Part model, mm, in its own coordinate system. A direction names the side the tool comes from. Round coordinates to 2 decimals unless told otherwise and drop trailing zeros. Order: outer loops, then holes, each group sorted by start corner. A loop starts at its lowest first (then second) coordinate and runs counter-clockwise, first axis right, second up. Notation, with made-up numbers: (11, -39.75) -> (36, -39.75) arc R27 cw to (36, -14.75) -> close; hole circle Ø8 at (29, 52). An arc over 180 degrees is marked (long way). Return JSON: item names as keys, results as strings. Group by question number.
from build123d import *

# Parameters (mm, degrees)
SKETCH1_W           = 42.3
SKETCH1_H           = 42.3
SKETCH1_R           = 2.5
BOSS_EXTRUDE1_DEPTH = 42.3
SKETCH2_R           = 2.5
BOSS_EXTRUDE2_DEPTH = 24
SKETCH3_R           = 7.5
BOSS_EXTRUDE3_DEPTH = 2
SKETCH4_W           = 15
SKETCH4_H           = 42.3
CUT_EXTRUDE1_DEPTH  = 1
SKETCH5_W           = 41.3
SKETCH5_H           = 15
CUT_EXTRUDE2_DEPTH  = 1


with BuildPart() as part:
    # Sketch1 → Boss-Extrude1 (new body)
    with BuildSketch(Plane.XY):
        Rectangle(SKETCH1_W, SKETCH1_H)
        with Locations((-15.5, 15.5)):
            Circle(SKETCH1_R, mode=Mode.SUBTRACT)
        with Locations((15.5, 15.5)):
            Circle(SKETCH1_R, mode=Mode.SUBTRACT)
        with Locations((15.5, -15.5)):
            Circle(SKETCH1_R, mode=Mode.SUBTRACT)
        with Locations((-15.5, -15.5)):
            Circle(SKETCH1_R, mode=Mode.SUBTRACT)
    extrude(amount=BOSS_EXTRUDE1_DEPTH)

    # Sketch2 → Boss-Extrude2 (add)
    with BuildSketch(Plane.XY.offset(42.3)):
        Circle(SKETCH2_R)
    extrude(amount=BOSS_EXTRUDE2_DEPTH)

    # Sketch3 → Boss-Extrude3 (add)
    with BuildSketch(Plane.XY.offset(42.3)):
        Circle(SKETCH3_R)
    extrude(amount=BOSS_EXTRUDE3_DEPTH)

    # Sketch4 → Cut-Extrude1 (cut)
    with BuildSketch(Plane(origin=(21.15, 0, 0), x_dir=(0, 0, -1), z_dir=(1, 0, 0))):
        with Locations((-21.15, 0)):
            Rectangle(SKETCH4_W, SKETCH4_H)
    cut_extrude1 = extrude(amount=-CUT_EXTRUDE1_DEPTH, mode=Mode.SUBTRACT)

    # Sketch5 → Cut-Extrude2 (cut)
    with BuildSketch(Plane(origin=(0, 21.15, 0), x_dir=(1, 0, 0), z_dir=(0, 1, 0))):
        with Locations((-0.5, -21.15)):
            Rectangle(SKETCH5_W, SKETCH5_H)
    extrude(amount=-CUT_EXTRUDE2_DEPTH, mode=Mode.SUBTRACT)

    # Mirror1: Cut-Extrude1 across plane
    add(cut_extrude1.mirror(Plane(origin=(0, 0, 0), x_dir=(0, 0, 1), z_dir=(1, 0, 0))), mode=Mode.SUBTRACT)


solid = part.part
(1) Saw through at C-C, the plane x = 14. List the corners of the cut face in (y, z), and give its area (3 significant figures).
(2) Pin check, flat tips, straight feed: P1, Ø4, axis at x = 15.5, y = -15.5, coming from the +Z side; P2, Ø4.5, axis at y = 5, z = 18.5, coming from the -X side; P3, Ø7.5, axis at x = 2, z = 20.5, coming from the +Y side; P4, Ø1, axis at x = 9, y = 7.5, coming from the +Z side. Stop position of each tip, or through.
(3) Tool access for faces 1 (the cylindrical face through (-7.493, 0.33, 43.286)), 2 (the flat face through (-21.15, 0, 7)): list every direction of +Z, -Z, +X, -X, +Y, -Y with a clear straight run to the whole face (end or side of a thin tool).
(4) Mould opens along Z. For faces 3 (the flat face through (0, 0, 0)), 4 (the flat face through (-0.1, 20.5, 13.65)), 5 (the cylindrical face through (-0.54, -2.44, 55.15)), 6 (the flat face through (20.15, 0, 21)) say: pulls with the +Z half, pulls with the -Z half, needs draft (parallel to the pull), parting line crosses it, or undercut.
(5) Saw through at D-D, the plane x = 0. List the corners of the cut face in (y, z).
(6) Saw through at B-B, the plane y = 15.5. List the corners of the cut face in (x, z).
(7) Saw through at A-A, the plane z = 32. List the corners of the cut face in (x, y), and give its area (3 significant figures).
(8) Probe L1, parallel to Y at x = -15.5, z = 17.5; L2, parallel to Y at x = -15, z = 17; L3, parallel to X at y = 15, z = 15. List the from-to ranges inside material, lowest first. Write a range as [from, to].
Results are:
{
 "1": {"outline": "(-21.15, 0) -> (-17.5, 0) -> (-17.5, 42.3) -> (-21.15, 42.3) -> close; (-13.5, 0) -> (13.5, 0) -> (13.5, 42.3) -> (-13.5, 42.3) -> close; (17.5, 0) -> (21.15, 0) -> (21.15, 13.65) -> (20.15, 13.65) -> (20.15, 28.65) -> (21.15, 28.65) -> (21.15, 42.3) -> (17.5, 42.3) -> close", "area": "1,440 mm^2"},
 "2": {"P1": "passes through", "P2": "stops at x = -20.15", "P3": "stops at y = 20.15", "P4": "stops at z = 42.3"},
 "3": {"face 1": "+Z", "face 2": "+Z, -Z, -X, +Y, -Y"},
 "4": {"face 3": "pulls with the -Z half", "face 4": "undercut", "face 5": "needs draft", "face 6": "undercut"},
 "5": {"outline": "(-21.15, 0) -> (21.15, 0) -> (21.15, 13.65) -> (20.15, 13.65) -> (20.15, 28.65) -> (21.15, 28.65) -> (21.15, 42.3) -> (7.5, 42.3) -> (7.5, 44.3) -> (2.5, 44.3) -> (2.5, 66.3) -> (-2.5, 66.3) -> (-2.5, 44.3) -> (-7.5, 44.3) -> (-7.5, 42.3) -> (-21.15, 42.3) -> close"},
 "6": {"outline": "(-21.15, 0) -> (-18, 0) -> (-18, 42.3) -> (-21.15, 42.3) -> (-21.15, 28.65) -> (-20.15, 28.65) -> (-20.15, 13.65) -> (-21.15, 13.65) -> close; (-13, 0) -> (13, 0) -> (13, 42.3) -> (-13, 42.3) -> close; (18, 0) -> (21.15, 0) -> (21.15, 13.65) -> (20.15, 13.65) -> (20.15, 28.65) -> (21.15, 28.65) -> (21.15, 42.3) -> (18, 42.3) -> close"},
 "7": {"outline": "(-21.15, -21.15) -> (21.15, -21.15) -> (21.15, 21.15) -> (-21.15, 21.15) -> close; hole circle Ø5 at (-15.5, -15.5); hole circle Ø5 at (-15.5, 15.5); hole circle Ø5 at (15.5, -15.5); hole circle Ø5 at (15.5, 15.5)", "area": "1,710 mm^2"},
 "8": {"L1": "y = [-21.15, -18], [-13, 13], [18, 20.15]", "L2": "y = [-21.15, -17.95], [-13.05, 13.05], [17.95, 20.15]", "L3": "x = [-20.15, -17.95], [-13.05, 13.05], [17.95, 20.15]"}
}
